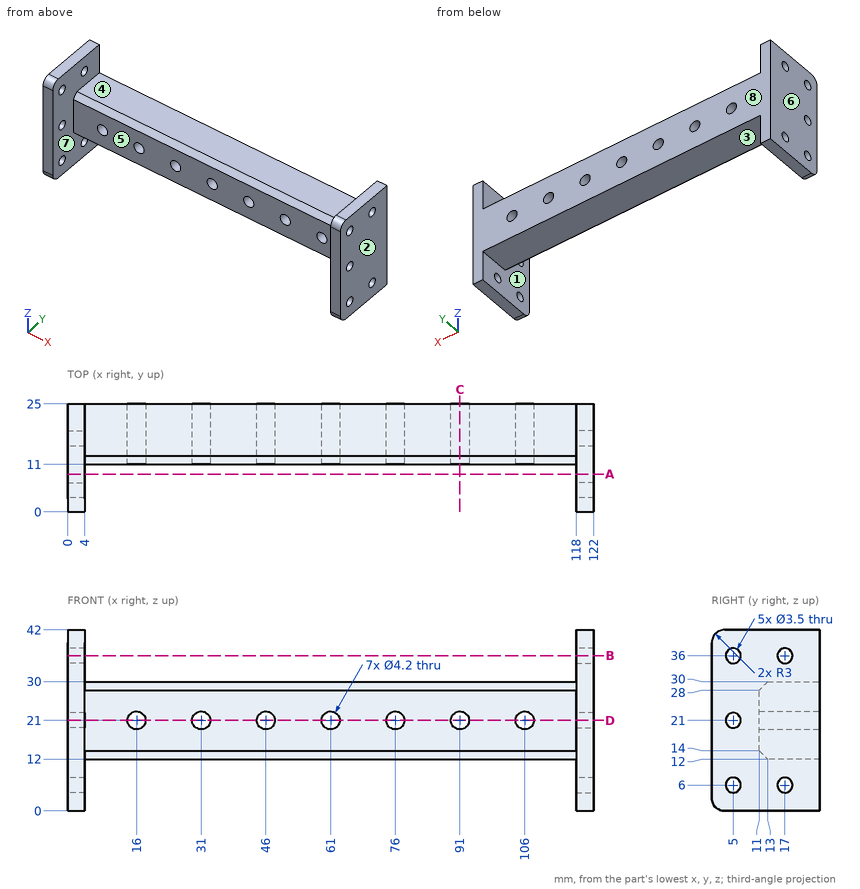
Design review of the part shown in the three views and the two pictorial views. Dimensions are in mm from the part's minimum x, y and z. A direction names the side the tool comes from. Give positions to 0.01 mm unless a question says otherwise; leave off trailing zeros. Write each loop counter-clockwise with the first axis right and the second up, starting at its lowest first coordinate (ties: lowest second). Pieces come first, ordered by that corner, then holes. Notation, with made-up numbers: M 82.25,-36.5 L 115.25,-36.5 A26 cw 115.25,-18.5 Z; hole C -7,38 d5. An arc over 180 degrees is marked long. Return JSON: item names as keys, results as strings. Group by question number.
Item 1: Clearance check with flat-ended pins moving along their axes: pin 1 Ø2 at (y, z) = (5, 21) entering from +X; pin 2 Ø10 at (x, y) = (80, 16) entering from -Z; pin 3 Ø1 at (x, y) = (82.5, 17) entering from +Z; pin 4 Ø5.5 at (x, z) = (61, 21) entering from -Y. State where each tip first meets the part, or that it passes through.
Item 2: Wall thickness on line 1 along Z through (x, y) = (0.9, 17); line 2 along Z through (x, y) = (31, 16.5); line 3 along X through (y, z) = (10.5, 19.5): over which ranges is each line inside the solid? List them lowest first.
Item 3: Take a section at A-A (y = 8.75). Give the boundary of the cut face in (x, z).
Item 4: Take a section at B-B (z = 36). Give the boundary of the cut face in (x, y), plus the area to 3 significant figures.
Item 5: Take a section at D-D (z = 21). Count the separate pieces of the cut face and the enclosed holes in it, plus the area to 3 significant figures.
Item 6: Tool access review of the marked faces 1, 2, 3, 4 and 5: name each direction out of +Z, -Z, +X, -X, +Y, -Y from which nothing blocks a thin tool from reaching the whole face with its end or side.
Item 7: Take a section at C-C (x = 91). Give the boundary of the cut face in (y, z).
Item 8: The part is to be moulded in two halves that separate along X. For the marked faces 6, 7 and 8, say which applies: pulls with the +X half, pulls with the -X half, needs draft (parallel to the pull), parting line crosses it, or undercut.
Return value:
{
 "1": {"pin 1": "passes through", "pin 2": "stops at z = 12", "pin 3": "stops at z = 30", "pin 4": "stops at y = 11"},
 "2": {"line 1": "z = 0 to 4.25, 7.75 to 34.25, 37.75 to 42", "line 2": "z = 12 to 18.9, 23.1 to 30", "line 3": "x = 0 to 4, 118 to 122"},
 "3": {"outline": "M 0,0 L 4,0 L 4,42 L 0,42 Z; M 118,0 L 122,0 L 122,42 L 118,42 Z"},
 "4": {"outline": "M 0,0 L 4,0 L 4,3.25 L 0,3.25 Z; M 0,6.75 L 4,6.75 L 4,15.25 L 0,15.25 Z; M 0,18.75 L 4,18.75 L 4,25 L 0,25 Z; M 118,0 L 122,0 L 122,3.25 L 118,3.25 Z; M 118,6.75 L 122,6.75 L 122,15.25 L 118,15.25 Z; M 118,18.75 L 122,18.75 L 122,25 L 118,25 Z", "area": "144 mm2"},
 "5": {"separate pieces": "10", "enclosed holes": "0", "area": "1,360 mm2"},
 "6": {"face 1": "-Y", "face 2": "+Z, -Z, +X, +Y, -Y", "face 3": "-Z, +Y, -Y", "face 4": "+Z, +Y, -Y", "face 5": "+Z, -Z, -Y"},
 "7": {"outline": "M 11,14 L 13,12 L 25,12 L 25,18.9 L 11,18.9 Z; M 11,23.1 L 25,23.1 L 25,30 L 13,30 L 11,28 Z"},
 "8": {"face 6": "pulls with the -X half", "face 7": "undercut", "face 8": "needs draft"}
}
